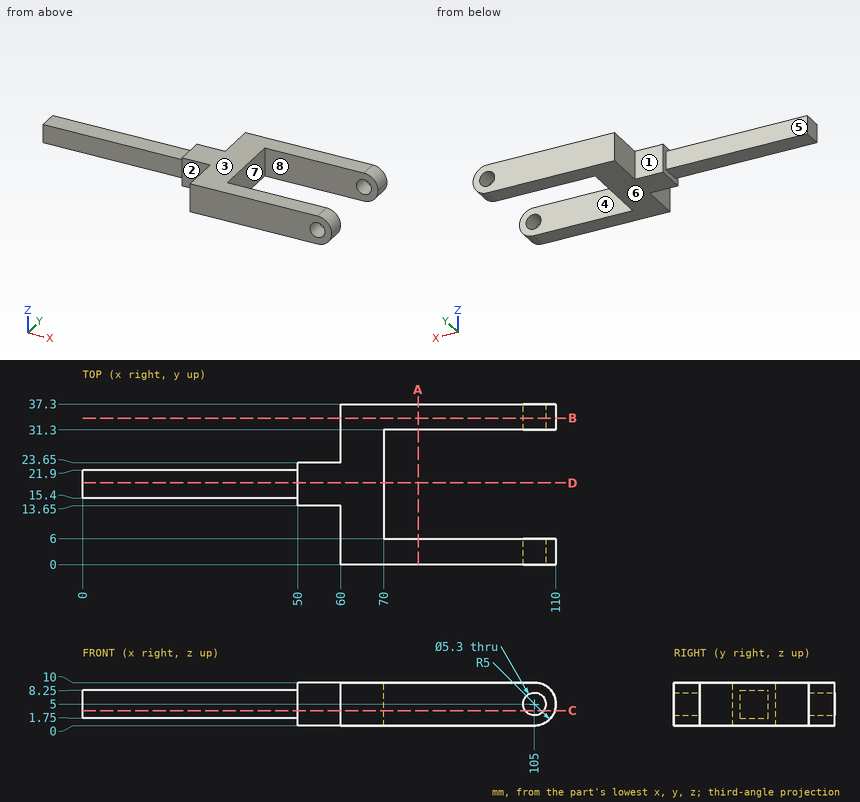
For this review, use the dimensioned drawing (mm, ordinates from the lowest corner) and the shaded views. A direction names the side the tool comes from. Round coordinates to 2 decimals unless told otherwise and drop trailing zeros. Write each loop counter-clockwise with the first axis right and the second up, starting at its lowest first coordinate (ties: lowest second). Pieces come first, ordered by that corner, then holes. Notation, with made-up numbers: M -7,79.5 L 21,79.5 A32 cw 21,117.5 Z; hole C -20,-25 d11. An arc over 180 degrees is marked long. Use CSV: the item, a comma, the result in double quotes. Start each with the question number.
(1) For line 1 along Y through (x, z) = (78, 7.25); line 2 along X through (y, z) = (32.9, 5); line 3 along Z through (x, y) = (105, 32.95), list the stretches that pass through material, from the lowest coordinate up.
(2) We need section D-D, the plane y = 19. State the section outline as (x, z) points.
(3) We need section A-A, the plane x = 78. State the section outline as (y, z) points.
(4) We need section C-C, the plane z = 3.5. State the section outline as (x, y) points, then the cut area to 3 significant figures.
(5) Clearance check with flat-ended pins moving along their axes: P1, Ø5, axis at y = 5, z = 6.5, coming from the -X side; P2, Ø3, axis at x = 17, y = 19, coming from the -Z side; P3, Ø3, axis at x = 56.5, z = 3, coming from the +Y side; P4, Ø5, axis at x = 87, z = 6, coming from the -Y side. State where each tip first meets the part, or that it passes through.
(6) We need section B-B, the plane y = 34. State the section outline as (x, z) points, then the cut area to 3 significant figures.
(7) Tool access review of the marked faces 1, 2, 3 and 4: name each direction out of +Z, -Z, +X, -X, +Y, -Y from which nothing blocks a thin tool from reaching the whole face with its end or side.
(8) The part is to be moulded in two halves that separate along Y. For the marked faces 5, 6, 7 and 8, say which applies: +Y half, -Y half, draft (parallel to the pull), parting line (faces both ways), or undercut.
Findings:
1,line 1,"0 to 6, 31.3 to 37.3"
1,line 2,"60 to 102.35, 107.65 to 110"
1,line 3,"0 to 2.35, 7.65 to 10"
2,outline,"M 0,1.75 L 50,1.75 L 50,0 L 70,0 L 70,10 L 50,10 L 50,8.25 L 0,8.25 Z"
3,outline,"M 0,0 L 6,0 L 6,10 L 0,10 Z; M 31.3,0 L 37.3,0 L 37.3,10 L 31.3,10 Z"
4,outline,"M 0,15.4 L 50,15.4 L 50,13.65 L 60,13.65 L 60,0 L 102.82,0 L 102.82,6 L 70,6 L 70,31.3 L 102.82,31.3 L 102.82,37.3 L 60,37.3 L 60,23.65 L 50,23.65 L 50,21.9 L 0,21.9 Z; M 107.18,0 L 109.77,0 L 109.77,6 L 107.18,6 Z; M 107.18,31.3 L 109.77,31.3 L 109.77,37.3 L 107.18,37.3 Z"
4,area,"1,220 mm^2"
5,P1,"x = 60"
5,P2,"z = 1.75"
5,P3,"y = 23.65"
5,P4,"y = 0"
6,outline,"M 60,0 L 105,0 A5 ccw 105,10 L 60,10 Z; hole C 105,5 d5.3"
6,area,"467 mm^2"
7,face 1,"+Z, -Z, -X, +Y"
7,face 2,"+Z, -Z, -X, -Y"
7,face 3,"+Z, +X, -X, +Y, -Y"
7,face 4,"+Z, -Z, +X"
8,face 5,"+Y half"
8,face 6,"draft"
8,face 7,"undercut"
8,face 8,"undercut"
